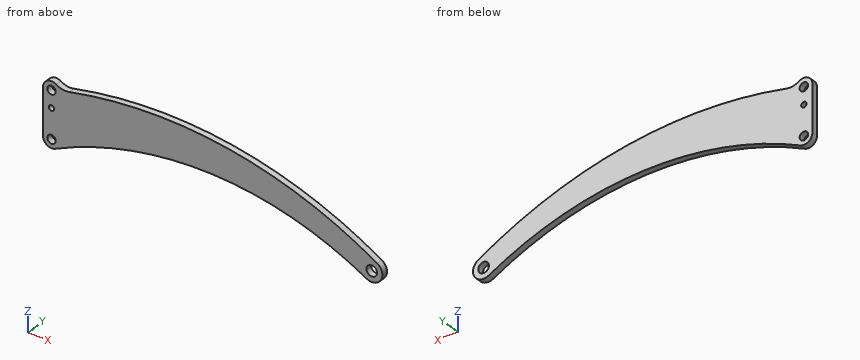
from build123d import *

# Parameters (mm, degrees)
F0_R     = 3.175
F0_R_2   = 3.96875
F0_R_3   = 1.984375
F1_DEPTH = 4.7625


with BuildPart() as f1:
    # F0 (on Front) → F1 (new body)
    with BuildSketch(Plane.XZ):
        with BuildLine():
            ThreePointArc((9.860095, 46.566667), (3.347218, 46.870159), (0, 41.275))
            Line((0, 41.275), (0, 6.35))
            ThreePointArc((0, 6.35), (2.964048, 0.978051), (9.089081, 0.621131))
            ThreePointArc((9.089081, 0.621131), (126.555864, 25.267368), (242.182661, -6.924648))
            ThreePointArc((242.182661, -6.924648), (252.929822, -3.980426), (250.142666, 6.808535))
            ThreePointArc((250.142666, 6.808535), (138.474992, 47.75611), (19.574735, 44.73912))
            ThreePointArc((19.574735, 44.73912), (14.532309, 44.668934), (9.860095, 46.566667))
        make_face()
        with Locations((6.35, 6.35)):
            Circle(F0_R, mode=Mode.SUBTRACT)
        with Locations((246.0625, 0)):
            Circle(F0_R_2, mode=Mode.SUBTRACT)
        with Locations((6.35, 28.575)):
            Circle(F0_R_3, mode=Mode.SUBTRACT)
        with Locations((6.35, 41.275)):
            Circle(F0_R, mode=Mode.SUBTRACT)
    extrude(amount=F1_DEPTH)


solid = f1.part
Design review of the part built by this model. Coordinates are the model's own, in mm. Round coordinates to 2 decimals unless told otherwise and drop trailing zeros. Write each loop counter-clockwise with the first axis right and the second up, starting at its lowest first coordinate (ties: lowest second). Pieces come first, ordered by that corner, then holes. Notation, with made-up numbers: (-25, -21.75) -> (1, -21.75) arc R7 ccw to (1, -16.75) -> close; hole circle Ø9 at (74.5, 84.5). An arc over 180 degrees is marked (long way). One line per question, with ' | ' between items.
(1) Take a section at A-A, the plane z = 12. State the section outline as (x, y) points.
Result sheet:
outline: (0, -4.76) -> (37.06, -4.76) -> (37.06, 0) -> (0, 0) -> close; (199.66, -4.76) -> (241.15, -4.76) -> (241.15, 0) -> (199.66, 0) -> close
(2) Take a section at D-D, the plane z = 36. State the section outline as (x, y) points.
Result sheet:
outline: (0, -4.76) -> (186.36, -4.76) -> (186.36, 0) -> (0, 0) -> close
(3) Take a section at B-B, the plane y = -3.05. State how many separate pieces and enclosed holes the cut face has, and give its area (3 significant figures).
Result sheet:
separate pieces: 1 | enclosed holes: 4 | area: 6,560 mm2
(4) Take a section at C-C, the plane x = 237.5. State the section outline as (y, z) points, and give its area (3 significant figures).
Result sheet:
outline: (-4.76, -4.37) -> (0, -4.37) -> (0, 14) -> (-4.76, 14) -> close | area: 87.4 mm2
(5) Insertion check: P1, Ø1, axis at x = 214.5, y = -1, coming from the +Z side; P2, Ø1, axis at y = -1, z = 12.5, coming from the +X side; P3, Ø1, axis at y = -1, z = 42.5, coming from the -X side. Each pin has a flat end and moves straight along its axis. Give the tip position at first contact, or say it passes through.
Result sheet:
P1: z = 25.43 | P2: x = 241.15 | P3: x = 0.04
(6) Wall thickness on line 1 (Z direction, x = 6.35, y = -1.3) (3 decimals); line 2 (X direction, y = -0.7, z = 1.5); line 3 (Z direction, x = 46, y = -3.65): over which ranges is each line inside the solid? List them lowest first. Write a range as [from, to].
Result sheet:
line 1: [0, 3.175], [9.525, 26.591], [30.559, 38.1], [44.45, 47.625] | line 2: [2.25, 10.95], [225.77, 242.39], [249.74, 253.86] | line 3: [14.85, 49.32]
